For this review, take the finished solid that the model builds, in its own axes (mm). Round coordinates to 2 decimals unless told otherwise and drop trailing zeros. Order: outer loops, then holes, each group sorted by start corner. A loop starts at its lowest first (then second) coordinate and runs counter-clockwise, first axis right, second up. Notation, with made-up numbers: (71.5, 16) - (106.5, 16) arc R31 cw to (106.5, 51) - close; hole circle Ø11 at (70, 84). An arc over 180 degrees is marked (long way). Write each question's results on one line, items separated by ' | '. Start each with the question number.
(1) Take a section at B-B, the plane x = 48. Give the boundary of the cut face in (y, z).
(2) For L1, parallel to X at y = 27, z = -125; L2, parallel to Z at x = 76, y = 15.5; L3, parallel to Z at x = -23, y = 4, list the stretches that pass through material, from the lowest coordinate up. Write a range as from..to.
(3) Draft analysis for pull direction Z (two halves, no side actions). For faces 1 (the flat face through (85, 20, 2.836)), 2 (the cylindrical face through (17.622, 35.944, -139.041)), 3 (the flat face through (13.709, 20, -124)), state which applies: pulls with the +Z half, pulls with the -Z half, needs draft (parallel to the pull), parting line crosses it, or undercut.
(4) Take a section at A-A, the plane y = 7.5. Give the number of separate pieces and of enclosed holes in the cut face, plus the area to 3 significant figures.
(5) Insertion check: pin 1 Ø0.9 at (y, z) = (25, -146) entering from +X; pin 2 Ø2.5 at (y, z) = (24, 1) entering from -X; pin 3 Ø3 at (x, z) = (-39.5, -121.5) entering from -Y; pin 4 Ø2.5 at (y, z) = (22, -145.5) entering from -X. Each pin has a flat end and moves straight along its axis. Give the tip position at first contact, or say it passes through.
(6) Take a section at C-C, the plane z = -131. Give the boundary of the cut face in (x, y), plus the area to 3 significant figures.
```python
from build123d import *

# Parameters (mm, degrees)
SKETCH8_W                      = 120
SKETCH8_H                      = 150
BOSS_EXTRUDE3_DEPTH            = 40
SKETCH9_R                      = 50
BOSS_EXTRUDE4_DEPTH            = 40
SHELL1_START                   = 3
SHELL1_DEPTH                   = 37
SKETCH17_R                     = 5
BOSS_EXTRUDE6_DEPTH            = 10
CUT_EXTRUDE9_DEPTH             = 203.818558951
CUT_EXTRUDE9_DEPTH_BACK        = 203.818558951
SKETCH11_W                     = 1.5
SKETCH11_H                     = 20
CUT_EXTRUDE10_DEPTH            = 205.88547515
CUT_EXTRUDE10_DEPTH_BACK       = 205.88547515
SKETCH12_W                     = 1.5
SKETCH12_H                     = 20
CUT_EXTRUDE11_DEPTH            = 203.818558951
CUT_EXTRUDE11_DEPTH_BACK       = 203.818558951
SKETCH15_W                     = 1.5
SKETCH15_H                     = 20
SKETCH28_R                     = 5
BOSS_EXTRUDE7_DEPTH            = 37
SKETCH29_R                     = 5
BOSS_EXTRUDE8_DEPTH            = 40
SKETCH30_R                     = 5
BOSS_EXTRUDE9_DEPTH            = 40
SKETCH31_R                     = 5
BOSS_EXTRUDE10_DEPTH           = 37
SKETCH32_R                     = 5
BOSS_EXTRUDE11_DEPTH           = 37
F_2_0_221_DIAMETER_HOLE1_D     = 5.6134
F_2_0_221_DIAMETER_HOLE1_DEPTH = 8
F_2_0_221_DIAMETER_HOLE1_TIP   = 1.686435499
F_2_0_221_DIAMETER_HOLE2_D     = 5.6134
F_2_0_221_DIAMETER_HOLE2_DEPTH = 8
F_2_0_221_DIAMETER_HOLE2_TIP   = 1.686435499
FILLET3_R                      = 4
FILLET2_R                      = 0.5


# Read off the part's stored shape, not the designer's step: Shell1
with BuildPart() as part:
    # Sketch8 → Boss-Extrude3 (new body)
    with BuildSketch(Plane(origin=(0, 0, 0), x_dir=(1, 0, 0), z_dir=(0, 1, 0))):
        with Locations((73.708855083, 72.164227744)):
            Rectangle(SKETCH8_W, SKETCH8_H)
    extrude(amount=BOSS_EXTRUDE3_DEPTH)

    # Sketch9 → Boss-Extrude4 (add)
    with BuildSketch(Plane(origin=(0, 0, 0), x_dir=(1, 0, 0), z_dir=(0, 1, 0))):
        with Locations((-22.779007595, 71.748458752)):
            Circle(SKETCH9_R)
    extrude(amount=BOSS_EXTRUDE4_DEPTH)

    # Shell1 outline → Shell1 (cut)
    with BuildSketch(Plane(origin=(0, 0, 0), x_dir=(1, 0, 0), z_dir=(0, 1, 0)).offset(SHELL1_START)):
        with BuildLine():
            Line((16.708855083, 46.259074664), (16.708855083, 0.164227744))
            Line((16.708855083, 0.164227744), (130.708855083, 0.164227744))
            Line((130.708855083, 0.164227744), (130.708855083, 144.164227744))
            Line((130.708855083, 144.164227744), (16.708855083, 144.164227744))
            Line((16.708855083, 144.164227744), (16.708855083, 97.237842839))
            ThreePointArc((16.708855083, 97.237842839), (-69.779007595, 71.748458751), (16.708855083, 46.259074664))
        make_face()
    extrude(amount=SHELL1_DEPTH, mode=Mode.SUBTRACT)

    # Sketch17 → Boss-Extrude6 (add)
    with BuildSketch(Plane(origin=(1.848761015, 3, -2.465014687), x_dir=(1, 0, 0), z_dir=(0, 1, 0))):
        with Locations(Location((111.867013496, 11.175325825, 0), (0, 0, 270))):
            Circle(SKETCH17_R)
        with Locations(Location((34.367013496, 11.175325825, 0), (0, 0, 270))):
            Circle(SKETCH17_R)
        with Locations(Location((111.867013496, 94.175325825, 0), (0, 0, 270))):
            Circle(SKETCH17_R)
        with Locations(Location((34.367013496, 94.175325825, 0), (0, 0, 270))):
            Circle(SKETCH17_R)
    extrude(amount=BOSS_EXTRUDE6_DEPTH)

    # Sketch11 → Cut-Extrude9 (cut, two sides: drawn at the far end of the back side and taken through both)
    with BuildSketch(Plane.XY.offset(-CUT_EXTRUDE9_DEPTH_BACK)):
        with Locations((73.491480368, 20.290686907)):
            Rectangle(SKETCH11_W, SKETCH11_H)
    extrude(amount=CUT_EXTRUDE9_DEPTH + CUT_EXTRUDE9_DEPTH_BACK, mode=Mode.SUBTRACT)

    # Sketch12 → Cut-Extrude10 (cut, two sides: drawn at the far end of the back side and taken through both)
    with BuildSketch(Plane.XY.offset(2.835772256).offset(-CUT_EXTRUDE10_DEPTH_BACK)):
        with Locations((77.588922832, 20.290686907)):
            Rectangle(SKETCH12_W, SKETCH12_H)
    extrude(amount=CUT_EXTRUDE10_DEPTH + CUT_EXTRUDE10_DEPTH_BACK, mode=Mode.SUBTRACT)

    # Sketch15 → Cut-Extrude11 (cut, two sides: drawn at the far end of the back side and taken through both)
    with BuildSketch(Plane.XY.offset(-CUT_EXTRUDE11_DEPTH_BACK)):
        with Locations((81.379057112, 20.290686907)):
            Rectangle(SKETCH15_W, SKETCH15_H)
    extrude(amount=CUT_EXTRUDE11_DEPTH + CUT_EXTRUDE11_DEPTH_BACK, mode=Mode.SUBTRACT)

    # Sketch28 → Boss-Extrude7 (add)
    with BuildSketch(Plane(origin=(0, 3, 0), x_dir=(1, 0, 0), z_dir=(0, 1, 0))):
        with Locations((19.708855083, 141.164227744)):
            Circle(SKETCH28_R)
    extrude(amount=BOSS_EXTRUDE7_DEPTH)

    # Sketch29 → Boss-Extrude8 (add)
    with BuildSketch(Plane(origin=(0, 0, 0), x_dir=(1, 0, 0), z_dir=(0, 1, 0))):
        with Locations((19.708855083, 3.164227744)):
            Circle(SKETCH29_R)
    extrude(amount=BOSS_EXTRUDE8_DEPTH)

    # Sketch30 → Boss-Extrude9 (add)
    with BuildSketch(Plane(origin=(0, 0, 0), x_dir=(1, 0, 0), z_dir=(0, 1, 0))):
        with Locations((127.708855083, 141.164227744)):
            Circle(SKETCH30_R)
    extrude(amount=BOSS_EXTRUDE9_DEPTH)

    # Sketch31 → Boss-Extrude10 (add)
    with BuildSketch(Plane(origin=(0, 3, 0), x_dir=(1, 0, 0), z_dir=(0, 1, 0))):
        with Locations((127.708855083, 3.164227744)):
            Circle(SKETCH31_R)
    extrude(amount=BOSS_EXTRUDE10_DEPTH)

    # Sketch32 → Boss-Extrude11 (add)
    with BuildSketch(Plane(origin=(0, 3, 0), x_dir=(1, 0, 0), z_dir=(0, 1, 0))):
        with Locations((-67.018543515, 71.628998297)):
            Circle(SKETCH32_R)
    extrude(amount=BOSS_EXTRUDE11_DEPTH)

    # #2 (0.221) Diameter Hole1
    with Locations(Plane(origin=(0, 40, 0), x_dir=(1, 0, 0), z_dir=(0, 1, 0))):
        with Locations((18.917123201, 141.531370062), (127.969984407, 141.269223761), (127.602547564, 3.45328248), (19.774147178, 3.570575466), (-67.115618064, 71.668740496)):
            Hole(F_2_0_221_DIAMETER_HOLE1_D / 2, depth=F_2_0_221_DIAMETER_HOLE1_DEPTH)
            with Locations((0, 0, -(F_2_0_221_DIAMETER_HOLE1_DEPTH + F_2_0_221_DIAMETER_HOLE1_TIP / 2))):  # 118° drill point
                Cone(0, F_2_0_221_DIAMETER_HOLE1_D / 2, F_2_0_221_DIAMETER_HOLE1_TIP, mode=Mode.SUBTRACT)

    # #2 (0.221) Diameter Hole2
    with Locations(Plane(origin=(0, 13, 0), x_dir=(1, 0, 0), z_dir=(0, 1, 0))):
        with Locations((113.866576204, 96.665654076), (36.269140625, 13.672370328), (113.866576204, 13.415425177), (36.224664422, 96.637257854)):
            Hole(F_2_0_221_DIAMETER_HOLE2_D / 2, depth=F_2_0_221_DIAMETER_HOLE2_DEPTH)
            with Locations((0, 0, -(F_2_0_221_DIAMETER_HOLE2_DEPTH + F_2_0_221_DIAMETER_HOLE2_TIP / 2))):  # 118° drill point
                Cone(0, F_2_0_221_DIAMETER_HOLE2_D / 2, F_2_0_221_DIAMETER_HOLE2_TIP, mode=Mode.SUBTRACT)

    # Fillet3
    fillet3_edges = [part.edges().sort_by_distance(p)[0] for p in [
        (13.708855083, 20, -147.164227744),
        (133.708855083, 20, -147.164227744),
        (133.708855083, 20, 2.835772256),
        (13.708855083, 20, 2.835772256),
    ]]
    fillet(fillet3_edges, radius=FILLET3_R)

    # Fillet2
    fillet2_edges = [part.edges().sort_by_distance(p)[0] for p in [
        (16.708855083, 21.5, -46.259074664),
        (16.708855083, 21.5, -97.237842839),
    ]]
    fillet(fillet2_edges, radius=FILLET2_R)


solid = part.part
```
Results below:
1) outline: (0, -147.16) - (40, -147.16) - (40, -144.16) - (3, -144.16) - (3, -0.16) - (40, -0.16) - (40, 2.84) - (0, 2.84) - close
2) L1: x = 13.71..16.71, 130.71..133.71 | L2: z = -147.16..-144.16, -0.16..2.84 | L3: z = -121.75..-118.75, -24.75..-21.75
3) face 1: pulls with the +Z half | face 2: undercut | face 3: needs draft
4) separate pieces: 5 | enclosed holes: 5 | area: 2,620 mm^2
5) pin 1: stops at x = 132.92 | pin 2: stops at x = 13.81 | pin 3: passes through | pin 4: stops at x = 13.86
6) outline: (13.71, 0) - (133.71, 0) - (133.71, 40) - (130.71, 40) - (130.71, 3) - (16.71, 3) - (16.71, 40) - (13.71, 40) - close | area: 582 mm^2
